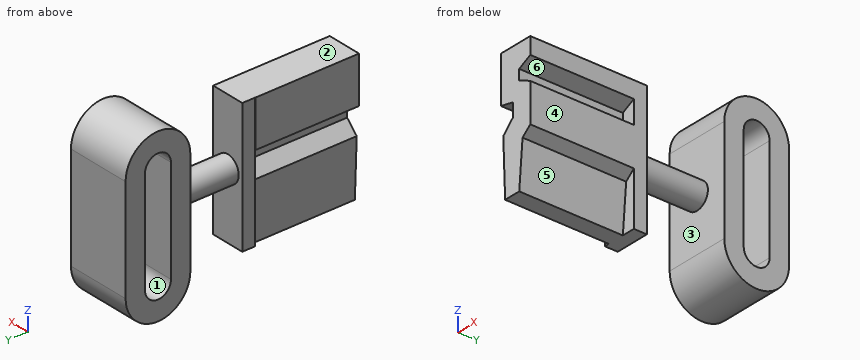
```python
from build123d import *

# Parameters (mm, degrees)
BOSS_EXTRUDE1_DEPTH = 8
SKETCH8_W           = 2.666068872
SKETCH8_H           = 10.16707981
BOSS_EXTRUDE2_DEPTH = 1
SKETCH9_R           = 1
BOSS_EXTRUDE3_DEPTH = 5
BOSS_EXTRUDE4_DEPTH = 2.5


with BuildPart() as part:
    # Sketch7 → Boss-Extrude1 (new body)
    with BuildSketch(Plane(origin=(0, 0, 0), x_dir=(1, 0, 0), z_dir=(0, 1, 0))):
        Polygon((-1.340563115, -5.083539905), (-1.340563115, -1.49622437), (-0.25317284, -1.264277343), (-0.25317284, -0.218468371), (-1.12873384, 0.657092629), (-0.958485867, 5.083539905), (0.330534493, 5.083539905), (0.634548729, 1.544814198), (1.340563115, 0.95051095), (1.340563115, -2.018232649), (0.330534493, -2.504655426), (0.330534493, -3.289882138), (1.340563115, -3.793675787), (1.340563115, -5.083539905), align=None)
    extrude(amount=-BOSS_EXTRUDE1_DEPTH)

    # Sketch8 → Boss-Extrude2 (add)
    with BuildSketch(Plane(origin=(0, 0, 0), x_dir=(1, 0, 0), z_dir=(0, 1, 0))):
        with Locations((0.007528679, 0)):
            Rectangle(SKETCH8_W, SKETCH8_H)
    extrude(amount=BOSS_EXTRUDE2_DEPTH)

    # Sketch9 → Boss-Extrude3 (add)
    with BuildSketch(Plane(origin=(0, 1, 0), x_dir=(1, 0, 0), z_dir=(0, 1, 0))):
        Circle(SKETCH9_R)
    extrude(amount=BOSS_EXTRUDE3_DEPTH)

    # Sketch11 → Boss-Extrude4 (add, symmetric)
    with BuildSketch(Plane(origin=(0, 0, 0), x_dir=(0, 0, -1), z_dir=(1, 0, 0))):
        with BuildLine():
            Line((-4, 11), (4, 11))
            ThreePointArc((4, 11), (6.5, 8.5), (4, 6))
            Line((4, 6), (-4, 6))
            ThreePointArc((-4, 6), (-6.5, 8.5), (-4, 11))
        make_face()
        with BuildLine():
            Line((-4, 9.5), (4, 9.5))
            ThreePointArc((4, 9.5), (5, 8.5), (4, 7.5))
            Line((4, 7.5), (-4, 7.5))
            ThreePointArc((-4, 7.5), (-5, 8.5), (-4, 9.5))
        make_face(mode=Mode.SUBTRACT)
    extrude(amount=BOSS_EXTRUDE4_DEPTH, both=True)


solid = part.part
```
CAD build for the part. Positions are in the model's coordinates, mm. Face numbers are marked on the shaded views. A direction names the side the tool comes from. Coordinates: 2 decimals unless noted, no trailing zeros. Write each loop counter-clockwise with the first axis right and the second up, starting at its lowest first coordinate (ties: lowest second). Pieces come first, ordered by that corner, then holes. Notation, with made-up numbers: (57.5, -21) -> (72.5, -21) arc R13 ccw to (72.5, -1) -> close; hole circle Ø4 at (88.25, 77). An arc over 180 degrees is marked (long way). Use CSV: the item, a comma, the result in double quotes. Start each with the question number.
Item 1: Two-plate mould, pull along Z, no slides. Class the marked faces 4, 5 and 6: +Z half, -Z half, draft (parallel to the pull), parting line (faces both ways), or undercut.
Item 2: Wall check: probe 1 along Y at (x, z) = (-1.65, 3.5); probe 2 along Y at (x, z) = (-0.45, 0.25); probe 3 along Y at (x, z) = (0.8, 3.25). Give the ranges that are in metal, low to high.
Item 3: Band-saw the part on D-D, the plane z = 0.5. Write the cut outline in (x, y).
Item 4: Band-saw the part on C-C, the plane x = 0. Write the cut outline in (y, z).
Item 5: Band-saw the part on B-B, the plane z = -2.25. Write the cut outline in (x, y), plus the area to 3 significant figures.
Item 6: Drop flat-ended pins along their axis: P1, Ø3, axis at x = 0.5, y = -3, coming from the +Z side; P2, Ø4, axis at y = -2.5, z = -5, coming from the -X side; P3, Ø0.8, axis at x = 1, z = -2.5, coming from the -Y side. Give the stop position or say it passes through.
Item 7: Band-saw the part on A-A, the plane y = 8.5. Write the cut outline in (x, z).
Item 8: Tool access for the marked faces 1, 2 and 3: list every direction of +Z, -Z, +X, -X, +Y, -Y with a clear straight run to the whole face (end or side of a thin tool).
Response values:
1,face 4,"draft"
1,face 5,"-Z half"
1,face 6,"undercut"
2,probe 1,"y = 6 to 7.5, 9.5 to 11"
2,probe 2,"y = 0 to 7.5, 9.5 to 11"
2,probe 3,"y = 0 to 1, 6 to 7.5, 9.5 to 11"
3,outline,"(-2.5, 6) -> (-0.87, 6) -> (-0.87, 1) -> (-1.33, 1) -> (-1.33, 0) -> (-0.25, 0) -> (-0.25, -8) -> (1.34, -8) -> (1.34, 1) -> (0.87, 1) -> (0.87, 6) -> (2.5, 6) -> (2.5, 7.5) -> (-2.5, 7.5) -> close; (-2.5, 9.5) -> (2.5, 9.5) -> (2.5, 11) -> (-2.5, 11) -> close"
4,outline,"(-8, -5.08) -> (1, -5.08) -> (1, -1) -> (6, -1) -> (6, -4) arc R2.5 ccw to (11, -4) -> (11, 4) arc R2.5 ccw to (6, 4) -> (6, 1) -> (1, 1) -> (1, 5.08) -> (-8, 5.08) -> close; hole (7.5, -4) arc R1 ccw to (9.5, -4) -> (9.5, 4) arc R1 ccw to (7.5, 4) -> close"
5,outline,"(-2.5, 6) -> (2.5, 6) -> (2.5, 7.5) -> (-2.5, 7.5) -> close; (-2.5, 9.5) -> (2.5, 9.5) -> (2.5, 11) -> (-2.5, 11) -> close; (-1.33, 0) -> (-1.07, 0) -> (-1.07, -8) -> (0.57, -8) -> (0.57, 0) -> (1.34, 0) -> (1.34, 1) -> (-1.33, 1) -> close"
5,area,"30.8 mm2"
6,P1,"stops at z = 5.08"
6,P2,"stops at x = -1.04"
6,P3,"stops at y = 0"
7,outline,"(-2.5, -6.5) -> (2.5, -6.5) -> (2.5, -5) -> (-2.5, -5) -> close; (-2.5, 5) -> (2.5, 5) -> (2.5, 6.5) -> (-2.5, 6.5) -> close"
8,face 1,"+X, -X"
8,face 2,"+Z, +X, -X, -Y"
8,face 3,"none"
